```python
from build123d import *

# Parameters (mm, degrees)
SKETCH1_W           = 207
SKETCH1_H           = 60
BOSS_EXTRUDE1_DEPTH = 5
SKETCH2_W           = 5
SKETCH2_H           = 15
CUT_EXTRUDE1_DEPTH  = 116.491341667
SKETCH3_W           = 167
SKETCH3_H           = 3
CUT_EXTRUDE2_DEPTH  = 5
SKETCH4_R           = 1.45
SKETCH4_R_2         = 1.95
SKETCH4_W           = 8
SKETCH4_H           = 2.9
SKETCH4_W_2         = 2.3
SKETCH4_H_2         = 5.35
SKETCH4_W_3         = 5.35
SKETCH4_H_3         = 2.3
SKETCH4_W_4         = 2.9
SKETCH4_H_4         = 8
CUT_EXTRUDE3_DEPTH  = 116.491341667


with BuildPart() as part:
    # Sketch1 → Boss-Extrude1 (new body)
    with BuildSketch(Plane.XY):
        with Locations((0, 21)):
            Rectangle(SKETCH1_W, SKETCH1_H)
    extrude(amount=BOSS_EXTRUDE1_DEPTH)

    # Sketch2 → Cut-Extrude1 (cut, through all)
    with BuildSketch(Plane.XY.offset(5)):
        with Locations((-101, 43.5)):
            Rectangle(SKETCH2_W, SKETCH2_H)
        with Locations((-101, -1.5)):
            Rectangle(SKETCH2_W, SKETCH2_H)
        with Locations((101, 43.5)):
            Rectangle(SKETCH2_W, SKETCH2_H)
        with Locations((101, -1.5)):
            Rectangle(SKETCH2_W, SKETCH2_H)
    extrude(amount=-CUT_EXTRUDE1_DEPTH, mode=Mode.SUBTRACT)

    # Sketch3 → Cut-Extrude2 (cut)
    with BuildSketch(Plane.XY.offset(5)):
        with Locations((0, 49.5)):
            Rectangle(SKETCH3_W, SKETCH3_H)
        with BuildLine():
            ThreePointArc((-81.5, -2), (-76.550252532, -4.050252532), (-74.5, -9))
            Line((-74.5, -9), (74.5, -9))
            ThreePointArc((74.5, -9), (76.550252532, -4.050252532), (81.5, -2))
            Line((81.5, -2), (-81.5, -2))
        make_face()
        with BuildLine():
            Line((-81.5, -2), (-81.5, -9))
            Line((-81.5, -9), (-74.5, -9))
            ThreePointArc((-74.5, -9), (-76.550252532, -4.050252532), (-81.5, -2))
        make_face()
        with BuildLine():
            Line((-88.5, -9), (-81.5, -9))
            Line((-81.5, -9), (-81.5, -2))
            ThreePointArc((-81.5, -2), (-86.449747468, -4.050252532), (-88.5, -9))
        make_face()
        with BuildLine():
            ThreePointArc((81.5, -2), (76.550252532, -4.050252532), (74.5, -9))
            Line((74.5, -9), (81.5, -9))
            Line((81.5, -9), (81.5, -2))
        make_face()
        with BuildLine():
            ThreePointArc((88.5, -9), (86.449747468, -4.050252532), (81.5, -2))
            Line((81.5, -2), (81.5, -9))
            Line((81.5, -9), (88.5, -9))
        make_face()
    extrude(amount=-CUT_EXTRUDE2_DEPTH, mode=Mode.SUBTRACT)

    # Sketch4 → Cut-Extrude3 (cut, through all)
    with BuildSketch(Plane.XY.offset(5)):
        with Locations((101, 23)):
            Circle(SKETCH4_R)
        with Locations((-101, 23)):
            Circle(SKETCH4_R)
        with Locations((-53.5, 9)):
            Circle(SKETCH4_R_2)
        with Locations((53.5, 9)):
            Circle(SKETCH4_R_2)
        with Locations((94.5, 43.5)):
            Rectangle(SKETCH4_W, SKETCH4_H)
        with Locations((94.5, -3)):
            Rectangle(SKETCH4_W, SKETCH4_H)
        with Locations((94.85, 43.5)):
            Rectangle(SKETCH4_W_2, SKETCH4_H_2)
        with Locations((94.85, -3)):
            Rectangle(SKETCH4_W_2, SKETCH4_H_2)
        with Locations((-94.85, -3)):
            Rectangle(SKETCH4_W_2, SKETCH4_H_2)
        with Locations((68.5, 44.35)):
            Rectangle(SKETCH4_W_3, SKETCH4_H_3)
        with Locations((68.5, 44)):
            Rectangle(SKETCH4_W_4, SKETCH4_H_4)
        with Locations((-94.5, 43.5)):
            Rectangle(SKETCH4_W, SKETCH4_H)
        with Locations((-94.85, 43.5)):
            Rectangle(SKETCH4_W_2, SKETCH4_H_2)
        with Locations((-94.5, -3)):
            Rectangle(SKETCH4_W, SKETCH4_H)
        with Locations((0, 44.35)):
            Rectangle(SKETCH4_W_3, SKETCH4_H_3)
        with Locations((0, 44)):
            Rectangle(SKETCH4_W_4, SKETCH4_H_4)
        with Locations((-68.5, 44)):
            Rectangle(SKETCH4_W_4, SKETCH4_H_4)
        with Locations((-68.5, 44.35)):
            Rectangle(SKETCH4_W_3, SKETCH4_H_3)
    extrude(amount=-CUT_EXTRUDE3_DEPTH, mode=Mode.SUBTRACT)


solid = part.part
```
For this review, take the finished solid that the model builds, in its own axes (mm). A direction names the side the tool comes from. Round coordinates to 2 decimals unless told otherwise and drop trailing zeros. Write each loop counter-clockwise with the first axis right and the second up, starting at its lowest first coordinate (ties: lowest second). Pieces come first, ordered by that corner, then holes. Notation, with made-up numbers: M -18,31 L 8,31 A13 cw 8,55 Z; hole C 78.25,-12.75 d10. An arc over 180 degrees is marked long. One line per item, written item: value. Start each with the question number.
(1) The part is to be moulded in two halves that separate along Y. For faces 6 (the flat face through (98.5, 2, 3)), 7 (the cylindrical face through (55.3, 8.25, 2.54)), 8 (the flat face through (77, 48, 3)), say which applies: released by +Y, released by -Y, zero draft, split by the parting line, or undercut.
(2) We need section B-B (z = 1.45). Count the separate pieces of the cut face and the enclosed holes in it, and give its area (3 significant figures).
(3) We need section D-D (x = -32). Give the boundary of the cut face in (y, z).
(4) We need section C-C (y = 3.5). Give the boundary of the cut face in (x, z), and give its area (3 significant figures).
(5) Wall thickness on line 1 (X direction, y = 41, z = 0.6); line 2 (Y direction, x = 53.5, z = 3.35); line 3 (Y direction, x = 101, z = 2.15): over which ranges is each line inside the solid? List them lowest first.
(6) We need section A-A (x = -53.5). Give the boundary of the cut face in (y, z), and give its area (4 significant figures).
(7) Insertion check: pin 1 (1 mm diameter, centred on y = 41.5, z = 1.5, fed in from -X); pin 2 (1 mm diameter, centred on y = -5, z = 2.5, fed in from +X); pin 3 (1 mm diameter, centred on x = 68, z = 4, fed in from -Y). Each pin has a flat end and moves straight along its axis. Give the tip position at first contact, or say it passes through.
(8) Machinability: for faces 1 (the flat face through (-98.5, -7, 3)), 2 (the cylindrical face through (86.5, -4.1, 2.5)), 3 (the flat face through (101, 6, 3)), 4 (the flat face through (101, 36, 3)), 5 (the flat face through (34, 48, 3)), which of the approach directions +Z, -Z, +X, -X, +Y, -Y give a long, thin tool a straight path to every point of the face, cutting with its end or side? Answer none if there is none.
Result:
1. face 6: zero draft
1. face 7: undercut
1. face 8: released by +Y
2. separate pieces: 1
2. enclosed holes: 4
2. area: 10,200 mm²
3. outline: M -2,0 L 48,0 L 48,5 L -2,5 Z
4. outline: M -98.5,0 L 98.5,0 L 98.5,5 L -98.5,5 Z
4. area: 985 mm²
5. line 1: -98.5 to -96, -93.7 to -69.95, -67.05 to -1.45, 1.45 to 67.05, 69.95 to 93.7, 96 to 98.5
5. line 2: -2 to 7.05, 10.95 to 48
5. line 3: 6 to 21.55, 24.45 to 36
6. outline: M -2,0 L 7.05,0 L 7.05,5 L -2,5 Z; M 10.95,0 L 48,0 L 48,5 L 10.95,5 Z
6. area: 230.5 mm²
7. pin 1: x = -98.5
7. pin 2: x = 98.5
7. pin 3: y = -2
8. face 1: +Z, -Z, -X, -Y
8. face 2: +Z, -Z, -Y
8. face 3: +Z, -Z, +X, -Y
8. face 4: +Z, -Z, +X, +Y
8. face 5: +Z, -Z, +Y
